For this review, take the finished solid that the model builds, in its own axes (mm). Face numbers are marked on the shaded views. A direction names the side the tool comes from. Give positions to 0.01 mm unless a question says otherwise; leave off trailing zeros. Write each loop counter-clockwise with the first axis right and the second up, starting at its lowest first coordinate (ties: lowest second). Pieces come first, ordered by that corner, then holes.
Q1. Machinability: for the marked faces 4, 5 and 6, which of the approach directions +Z, -Z, +X, -X, +Y, -Y give a long, thin tool a straight path to every point of the face, cutting with its end or side? Answer none if there is none.
Q2. We need section C-C (x = 34). Write out the cut boundary in (y, z).
Q3. For line 1 (X direction, y = -65.3, z = 3.5) (3 decimals); line 2 (X direction, y = -65.8, z = 3.5) (3 decimals); line 3 (Y direction, x = -7.6, z = 3.5), list the stretches that pass through material, from the lowest coordinate up.
Q4. We need section B-B (x = -0.5). Write out the cut boundary in (y, z), then the cut area to 3 significant figures.
Q5. We need section A-A (z = 3.5). Give the number of separate pieces and of enclosed holes in the cut face, then the cut area to 3 significant figures.
Q6. Insertion check: P1, Ø4, axis at y = -6, z = 1.5, coming from the -X side; P2, Ø3.5, axis at x = 48, z = 2.5, coming from the +Y side; P3, Ø2, axis at y = 2, z = 5, coming from the +X side. Each pin has a flat end and moves straight along its axis. Give the tip position at first contact, or say it passes through.
Q7. Mouldability with a two-part tool opening along X and no side actions: class the marked faces 1, 2 and 3 as released by +X, released by -X, zero draft, split by the parting line, or undercut.
```python
from build123d import *

# Parameters (mm, degrees)
SALIENTE_EXTRUIR3_DEPTH    = 7
CORTAR_EXTRUIR2_DEPTH      = 86.560604398
CORTAR_EXTRUIR2_DEPTH_BACK = 86.560604398
CROQUIS5_R                 = 1.5
CROQUIS6_R                 = 1.65
SALIENTE_EXTRUIR4_DEPTH    = 15
CROQUIS7_W                 = 6.07
CROQUIS7_H                 = 7
CORTAR_EXTRUIR3_DEPTH      = 86.560604398
CROQUIS8_W                 = 36.455
CROQUIS8_H                 = 4
CORTAR_EXTRUIR4_DEPTH      = 86.560604398


with BuildPart() as part:
    # Croquis4 → Saliente-Extruir3 (new body)
    with BuildSketch(Plane.XY):
        Polygon((-38.847108579, -68), (-10.628441913, -4), (-15, -4), (-41.455, -64), (-51.455, -64), (-51.455, -68), align=None)
        Polygon((0, -4), (0, 0), (-51.455, 0), (-51.455, -4), (-15, -4), (-10.628441913, -4), align=None)
        Polygon((51.455, -4), (51.455, 0), (0, 0), (0, -4), (10.628441913, -4), (15, -4), align=None)
        Polygon((41.455, -64), (15, -4), (10.628441913, -4), (38.847108579, -68), (51.455, -68), (51.455, -64), align=None)
    extrude(amount=SALIENTE_EXTRUIR3_DEPTH)

    # Croquis5 → Cortar-Extruir2 (cut, two sides: drawn at the far end of the back side and taken through both)
    with BuildSketch(Plane(origin=(0, 0, 0), x_dir=(1, 0, 0), z_dir=(0, 1, 0)).offset(-CORTAR_EXTRUIR2_DEPTH_BACK)):
        with Locations(Location((-47.525, -3.5, 0), (0, 0, 180))):
            Circle(CROQUIS5_R)
        with Locations(Location((47.525, -3.5, 0), (0, 0, 180))):
            Circle(CROQUIS5_R)
    extrude(amount=CORTAR_EXTRUIR2_DEPTH + CORTAR_EXTRUIR2_DEPTH_BACK, mode=Mode.SUBTRACT)

    # Croquis6 → Saliente-Extruir4 (add, symmetric)
    with BuildSketch(Plane(origin=(0, 0, 0), x_dir=(0, 0, -1), z_dir=(1, 0, 0))):
        with BuildLine():
            Line((-7, 0), (0, 0))
            Line((0, 0), (0, 3.5))
            ThreePointArc((0, 3.5), (-3.5, 7), (-7, 3.5))
            Line((-7, 3.5), (-7, 0))
        make_face()
        with Locations((-3.5, 3.5)):
            Circle(CROQUIS6_R, mode=Mode.SUBTRACT)
    extrude(amount=SALIENTE_EXTRUIR4_DEPTH, both=True)

    # Croquis7 → Cortar-Extruir3 (cut, through all)
    with BuildSketch(Plane.XY.offset(7)):
        with Locations((-11.965, 3.5)):
            Rectangle(CROQUIS7_W, CROQUIS7_H)
        with Locations((11.965, 3.5)):
            Rectangle(CROQUIS7_W, CROQUIS7_H)
        with Locations((0, 3.5)):
            Rectangle(CROQUIS7_W, CROQUIS7_H)
    extrude(amount=-CORTAR_EXTRUIR3_DEPTH, mode=Mode.SUBTRACT)

    # Croquis8 → Cortar-Extruir4 (cut, through all)
    with BuildSketch(Plane.XY.offset(7)):
        with Locations((-33.2275, -2)):
            Rectangle(CROQUIS8_W, CROQUIS8_H)
        with Locations((33.2275, -2)):
            Rectangle(CROQUIS8_W, CROQUIS8_H)
    extrude(amount=-CORTAR_EXTRUIR4_DEPTH, mode=Mode.SUBTRACT)


solid = part.part
```
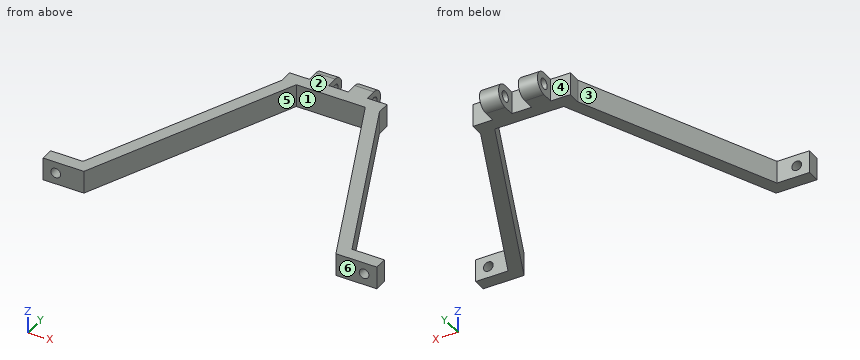
Computed:
1. face 4: +Z, -Z, -X, +Y
1. face 5: +Z, -Z, -Y
1. face 6: +Z, -Z, +X, -X, -Y
2. outline: (-57.01, 0) - (-47.09, 0) - (-47.09, 7) - (-57.01, 7) - close
3. line 1: x = -51.455 to -49.025, -46.025 to -37.657, 37.657 to 46.025, 49.025 to 51.455
3. line 2: x = -51.455 to -49.025, -46.025 to -37.877, 37.877 to 46.025, 49.025 to 51.455
3. line 3: y = -4 to 1.85, 5.15 to 7
4. outline: (-4, 0) - (0, 0) - (0, 7) - (-4, 7) - close
4. area: 28.0 mm2
5. separate pieces: 5
5. enclosed holes: 0
5. area: 772 mm2
6. P1: stops at x = -16.76
6. P2: stops at y = -64
6. P3: stops at x = 8.93
7. face 1: undercut
7. face 2: zero draft
7. face 3: released by -X
